Can you work these out from the model? Positions are in its coordinate system, mm. Face numbers are marked on the shaded views. A direction names the side the tool comes from. Coordinates: 2 decimals unless noted, no trailing zeros. Write each loop counter-clockwise with the first axis right and the second up, starting at its lowest first coordinate (ties: lowest second). Pieces come first, ordered by that corner, then holes. Notation, with made-up numbers: M 16.5,51 L 42.5,51 A27 cw 42.5,89 Z; hole C -24,-30.75 d3. An arc over 180 degrees is marked long. Use one line per item in the form item = value. Start each with the question number.
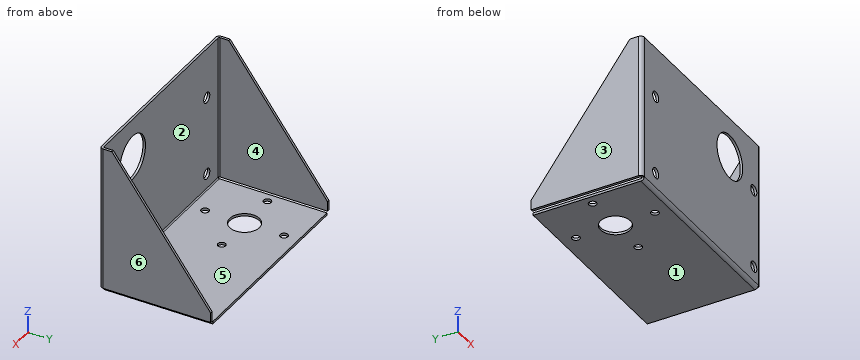
```python
from build123d import *

# Parameters (mm, degrees)
BASE_FLANGE1_DEPTH           = 127
EDGE_FLANGE1_DEPTH           = 92.9259
EDGE_FLANGE1_START           = 1.5875
EDGE_FLANGE1_FLAT_DEPTH      = 1.5875
EDGE_FLANGE1_BEND_DEPTH      = 92.9259
EDGE_FLANGE1_FLAT_2_DEPTH    = 1.5875
SKETCH15_R                   = 14.2875
CUT_EXTRUDE1_DEPTH           = 176.146532483
SKETCH16_R                   = 3.3782
CUT_EXTRUDE2_DEPTH           = 176.146532483
SKETCH17_R                   = 9.525
CUT_EXTRUDE3_DEPTH           = 175.288293488
F_10_0_1935_DIAMETER_HOLE1_D = 4.9149


# Sheet-metal steps are written as plain solids
with BuildPart() as part:
    # Sketch1 → Base-Flange1 (new body)
    with BuildSketch(Plane(origin=(0, 0, 0), x_dir=(0, 0, -1), z_dir=(1, 0, 0))):
        with BuildLine():
            Line((0, 0), (92.9259, 0))
            ThreePointArc((92.9259, 0), (93.446754855, 0.215745145), (93.6625, 0.7366))
            Line((93.6625, 0.7366), (93.6625, 69.85))
            Line((93.6625, 69.85), (95.25, 69.85))
            Line((95.25, 69.85), (95.25, 0.7366))
            ThreePointArc((95.25, 0.7366), (94.56928687, -0.90678687), (92.9259, -1.5875))
            Line((92.9259, -1.5875), (0, -1.5875))
            Line((0, -1.5875), (0, 0))
        make_face()
    extrude(amount=BASE_FLANGE1_DEPTH)

    # Edge-Flange1 bend section (across the edge) → Edge-Flange1 (add)
    with BuildSketch(Plane(origin=(-0.7366, 0, -92.9259), x_dir=(1, 0, 0), z_dir=(0, 0, 1))):
        with BuildLine():
            Line((-1.5875, 0.7366), (0, 0.7366))
            ThreePointArc((0, 0.7366), (0.215745145, 0.215745145), (0.7366, 0))
            Line((0.7366, 0), (0.7366, -1.5875))
            ThreePointArc((0.7366, -1.5875), (-0.90678687, -0.90678687), (-1.5875, 0.7366))
        make_face()
    extrude(amount=EDGE_FLANGE1_DEPTH)

    # Edge-Flange1 profile (on flange) → Edge-Flange1 flat (add)
    with BuildSketch(Plane.ZY.offset(0.7366).offset(EDGE_FLANGE1_START)):
        Polygon((0, 0.7366), (0, 6.35), (-86.5759, 69.85), (-92.9259, 69.85), (-92.9259, 0.7366), align=None)
    extrude(amount=-EDGE_FLANGE1_FLAT_DEPTH)

    # Edge-Flange1 bend section 2 (across the edge) → Edge-Flange1 bend (add)
    with BuildSketch(Plane(origin=(127.7366, 0, 0), x_dir=(-1, 0, 0), z_dir=(0, 0, -1))):
        with BuildLine():
            Line((-1.5875, 0.7366), (0, 0.7366))
            ThreePointArc((0, 0.7366), (0.215745145, 0.215745145), (0.7366, 0))
            Line((0.7366, 0), (0.7366, -1.5875))
            ThreePointArc((0.7366, -1.5875), (-0.90678687, -0.90678687), (-1.5875, 0.7366))
        make_face()
    extrude(amount=EDGE_FLANGE1_BEND_DEPTH)

    # Edge-Flange1 profile 2 (on flange) → Edge-Flange1 flat 2 (add)
    with BuildSketch(Plane(origin=(127.7366, 0, 0), x_dir=(0, 0, -1), z_dir=(1, 0, 0)).offset(EDGE_FLANGE1_START)):
        Polygon((0, 6.35), (0, 0.7366), (92.9259, 0.7366), (92.9259, 69.85), (86.5759, 69.85), align=None)
    extrude(amount=-EDGE_FLANGE1_FLAT_2_DEPTH)

    # Sketch15 → Cut-Extrude1 (cut, through all)
    with BuildSketch(Plane(origin=(0, 0, 0), x_dir=(1, 0, 0), z_dir=(0, 1, 0))):
        with Locations(Location((95.25, 25.4, 0), (0, 0, 270))):
            Circle(SKETCH15_R)
    extrude(amount=-CUT_EXTRUDE1_DEPTH, mode=Mode.SUBTRACT)

    # Sketch16 → Cut-Extrude2 (cut, through all)
    with BuildSketch(Plane(origin=(0, 0, 0), x_dir=(1, 0, 0), z_dir=(0, 1, 0))):
        with Locations(Location((12.7, 83.4009, 0), (0, 0, 270))):
            Circle(SKETCH16_R)
        with Locations(Location((121.92, 83.4009, 0), (0, 0, 270))):
            Circle(SKETCH16_R)
        with Locations(Location((121.92, 32.6009, 0), (0, 0, 270))):
            Circle(SKETCH16_R)
        with Locations(Location((12.7, 32.6009, 0), (0, 0, 270))):
            Circle(SKETCH16_R)
    extrude(amount=-CUT_EXTRUDE2_DEPTH, mode=Mode.SUBTRACT)

    # Sketch17 → Cut-Extrude3 (cut, through all)
    with BuildSketch(Plane.XY.offset(-93.6625)):
        with Locations((31.75, 35.2933)):
            Circle(SKETCH17_R)
    extrude(amount=-CUT_EXTRUDE3_DEPTH, mode=Mode.SUBTRACT)

    # #10 (0.1935) Diameter Hole1 (through all)
    with Locations(Plane(origin=(0, 0, -95.25), x_dir=(-1, 0, 0), z_dir=(0, 0, -1))):
        with Locations((-31.75, 60.6933), (-6.35, 35.2933), (-31.75, 9.8933), (-57.15, 35.2933)):
            Hole(F_10_0_1935_DIAMETER_HOLE1_D / 2)


solid = part.part
```
1) Suppose I cut it at A-A on x = 95.25. Please give me the cut outline in (y, z).
2) Please list where these lines run through material, in increasing order: line 1 (X direction, y = 22.5, z = -33); line 2 (Y direction, x = 31, z = -94); line 3 (Y direction, x = 31.5, z = -17).
3) Will these pins go through, and if not, where does the flat tip stop? pin 1 Ø1.9 at (x, y) = (128.5, 45.5) entering from -Z; pin 2 Ø2 at (x, z) = (49, -58.5) entering from +Y; pin 3 Ø4 at (x, y) = (57.15, 35.29) entering from -Z; pin 4 Ø6.5 at (x, y) = (31.75, 9.89) entering from +Z.
4) Suppose I cut it at D-D on y = 42. Please give me the cut outline in (x, z), and give its area (3 significant figures).
5) Which directions (+Z, -Z, +X, -X, +Y, -Y) give clear straight access to the entire face, cutting with the end or side of a thin tool? Please do the marked faces 4, 5 and 6.
6) Suppose I cut it at B-B on y = 4. Please give me the cut outline in (x, z).
7) Suppose I cut it at C-C on x = 121.92. Please give me the cut outline in (y, z), and give its area (3 significant figures).
8) If we mould it in two halves opening along X, with no side actions, what happens to the marked faces 1, 2 and 3? For each: +X half, -X half, draft (parallel to the pull), parting line (faces both ways), or undercut.
Computed values:
q1.outline = M -1.59,-92.93 A2.32 ccw 0.74,-95.25 L 69.85,-95.25 L 69.85,-93.66 L 0.74,-93.66 A0.74 cw 0,-92.93 L 0,-39.69 L -1.59,-39.69 Z; M -1.59,-11.11 L 0,-11.11 L 0,0 L -1.59,0 Z
q2.line_1 = -2.32 to -0.74, 127.74 to 129.32
q2.line_2 = -1.32 to 7.55, 12.23 to 25.8, 44.79 to 58.35, 63.03 to 69.85
q2.line_3 = -1.59 to 0
q3.pin_1 = -92.93
q3.pin_2 = 0
q3.pin_3 = through
q3.pin_4 = -93.66
q4.outline = M -2.32,-92.93 L -0.74,-92.93 L -0.74,-48.61 L -2.32,-48.61 Z; M 0,-95.25 L 24.99,-95.25 L 24.99,-93.66 L 0,-93.66 Z; M 38.51,-95.25 L 127,-95.25 L 127,-93.66 L 38.51,-93.66 Z; M 127.74,-92.93 L 129.32,-92.93 L 129.32,-48.61 L 127.74,-48.61 Z
q4.area = 321 mm²
q5.face_4 = +Z, -Z, +Y
q5.face_5 = +Z, +X, -X, +Y
q5.face_6 = +Z, -Z, +X, +Y, -Y
q6.outline = M -2.32,-92.93 L -0.74,-92.93 L -0.74,0 L -2.32,0 Z; M 0,-95.25 L 127,-95.25 L 127,-93.66 L 0,-93.66 Z; M 127.74,-92.93 L 129.32,-92.93 L 129.32,0 L 127.74,0 Z
q7.outline = M -1.59,-92.93 A2.32 ccw 0.74,-95.25 L 69.85,-95.25 L 69.85,-93.66 L 0.74,-93.66 A0.74 cw 0,-92.93 L 0,-86.78 L -1.59,-86.78 Z; M -1.59,-80.02 L 0,-80.02 L 0,-35.98 L -1.59,-35.98 Z; M -1.59,-29.22 L 0,-29.22 L 0,0 L -1.59,0 Z
q7.area = 240 mm²
q8.face_1 = draft
q8.face_2 = undercut
q8.face_3 = -X half
